The listing builds one solid part. Answer for the finished solid, in the listing's coordinates (mm). A direction names the side the tool comes from. Give positions to 0.01 mm unless a question says otherwise; leave off trailing zeros. Loops run counter-clockwise (first coordinate to the right, second up) from the corner with the lowest first, then second, coordinate; pieces in that order, holes last.
Item 1: Consider line 1 along X through (y, z) = (0.75, -61.5); line 2 along Y through (x, z) = (24, -152.5); line 3 along X through (y, z) = (6, -70). Determine where each line is inside the solid, lowest interval first.
Item 2: A tool of negligible diameter and unlimited length cuts with its end or side. For faces 1 (the face through (16.4, 3.1, 0)), 2 (the face through (24, -2.886, -164)), 3 (the face through (0.834, 4.565, -164.354)), from which of +Z, -Z, +X, -X, +Y, -Y can it reach the whole face along a straight path? Write none if from no direction.
Item 3: Each of these flat-tipped pins is pushed along its axis until it touches: pin 1 Ø1.5 at (y, z) = (6.5, -200) entering from -X; pin 2 Ø1 at (x, z) = (25, -272) entering from +Y; pin 3 Ø0.6 at (y, z) = (1, -230.5) entering from -X; pin 4 Ø5 at (x, y) = (10, 3.5) entering from +Z. Where does it stop, or does it pass through?
Item 4: Section C-C, the plane x = 6.5 is taken. Give the vertices of the cut face in (y, z) (3 decimals), and give its area (3 significant figures).
Item 5: Section B-B, the plane z = -219 is taken. Give the vertices of the cut face in (x, y), and give its area (3 significant figures).
Item 6: The mould has two halves that part along Y. Classify faces 4 (the face through (16.4, 3.1, -333.375)), 5 (the face through (25, -3.902, -164)), 6 (the face through (19.011, 1.874, -164.354)): pulls with the +Y half, pulls with the -Y half, needs draft (parallel to the pull), parting line crosses it, or undercut.
Item 7: Section A-A, the plane x = 21 is taken. Give the vertices of the cut face in (y, z) (3 decimals).
from build123d import *

# Parameters (mm, degrees)
EXTRUDE_THIN1_DEPTH = 333.375
FILLET1_R           = 1.016


with BuildPart() as part:
    # Sketch1 → Extrude-Thin1 (new body)
    with BuildSketch(Plane.XY):
        with BuildLine():
            Line((0, 0), (-0.396875, 9.921875))
            ThreePointArc((-0.396875, 9.921875), (6.530313151, 9.224476066), (12.744287778, 6.084600226))
            ThreePointArc((12.744287778, 6.084600226), (19.730938199, 2.736608506), (27.472950555, 2.44751107))
            Line((27.472950555, 2.44751107), (27.472950555, 0.06626107))
            Line((27.472950555, 0.06626107), (32.940625, -0.72748893))
            Line((32.940625, -0.72748893), (32.940625, -3.90248893))
            Line((32.940625, -3.90248893), (17.065625, -3.90248893))
            Line((17.065625, -3.90248893), (17.065625, -2.88648893))
            Line((17.065625, -2.88648893), (31.924625, -2.88648893))
            Line((31.924625, -2.88648893), (31.924625, -1.606644926))
            Line((31.924625, -1.606644926), (26.456950555, -0.812894926))
            Line((26.456950555, -0.812894926), (26.456950555, 1.28155123))
            ThreePointArc((26.456950555, 1.28155123), (18.908627692, 1.902340806), (12.12809243, 5.276788804))
            ThreePointArc((12.12809243, 5.276788804), (6.71021132, 8.106692295), (0.658241432, 8.964276082))
            Line((0.658241432, 8.964276082), (1.015188174, 0.040607527))
            Line((1.015188174, 0.040607527), (0, 0))
        make_face()
    extrude(amount=-EXTRUDE_THIN1_DEPTH)

    # Fillet1
    fillet1_edges = [part.edges().sort_by_distance(p)[0] for p in [
        (26.456950555, -0.812894926, -166.6875),
        (-0.396875, 9.921875, -166.6875),
        (27.472950555, 2.44751107, -166.6875),
        (32.940625, -0.72748893, -166.6875),
        (32.940625, -3.90248893, -166.6875),
    ]]
    fillet(fillet1_edges, radius=FILLET1_R)


solid = part.part
Worked answers:
1. line 1: x = -0.03 to 0.99, 26.46 to 27.47
1. line 2: y = -3.9 to -2.89, 1.17 to 2.18
1. line 3: x = -0.24 to 0.78, 11.11 to 12.86
2. face 1: +Z, +X, -X, +Y, -Y
2. face 2: +Z, -Z, -X
2. face 3: +Z, -Z
3. pin 1: stops at x = -0.29
3. pin 2: stops at y = 2.22
3. pin 3: stops at x = -0.05
3. pin 4: passes through
4. outline: (8.173, -333.375) - (9.233, -333.375) - (9.233, 0) - (8.173, 0) - close
4. area: 354 mm2
5. outline: (-0.36, 8.92) - (0, 0) - (1.02, 0.04) - (0.66, 8.96) arc R18.03 cw to (12.13, 5.28) arc R20.07 ccw to (26.46, 1.28) - (26.46, 0.07) arc R1.02 ccw to (27.33, -0.94) - (31.92, -1.61) - (31.92, -2.89) - (17.07, -2.89) - (17.07, -3.9) - (31.92, -3.9) arc R1.02 ccw to (32.94, -2.89) - (32.94, -1.61) arc R1.02 ccw to (32.07, -0.6) - (27.47, 0.07) - (27.47, 1.28) arc R1.02 ccw to (26.35, 2.29) arc R19.05 cw to (12.74, 6.08) arc R19.05 ccw to (0.63, 9.98) arc R1.02 ccw to start
5. area: 63.3 mm2
6. face 4: needs draft
6. face 5: pulls with the -Y half
6. face 6: undercut
7. outline: (-3.902, -333.375) - (-2.886, -333.375) - (-2.886, 0) - (-3.902, 0) - close; (1.438, -333.375) - (2.469, -333.375) - (2.469, 0) - (1.438, 0) - close
